```python
from build123d import *

# Parameters (mm, degrees)
F0_W     = 101.6
F0_H     = 50.8
F1_DEPTH = 25.4
F2_W     = 50.8
F2_H     = 12.7
F3_DEPTH = 25.401
F4_W     = 19.05
F4_H     = 12.7
F5_DEPTH = 25.401
F6_R     = 6.35
F7_DEPTH = 50.801
F8_DEPTH = 50.801


with BuildPart() as f1:
    # F0 (on Front) → F1 (new body)
    with BuildSketch(Plane.XZ):
        Rectangle(F0_W, F0_H)
    extrude(amount=F1_DEPTH)

    # F2 (on face) → F3 (cut, through all)
    with BuildSketch(Plane.XZ.offset(25.4)):
        with Locations((0, 19.05)):
            Rectangle(F2_W, F2_H)
    extrude(amount=-F3_DEPTH, mode=Mode.SUBTRACT)

    # F4 (on Front) → F5 (cut, through all)
    with BuildSketch(Plane.XZ):
        with Locations((41.358551, -19.152182)):
            Rectangle(F4_W, F4_H)
    extrude(amount=F5_DEPTH, mode=Mode.SUBTRACT)

    # F6 (on Right) → F7 (cut, through all)
    with BuildSketch(Plane.YZ):
        with Locations((-13.521904, 0.013301)):
            Circle(F6_R)
    extrude(amount=-F7_DEPTH, mode=Mode.SUBTRACT)

    # F6 (on Right) → F8 (cut, through all)
    with BuildSketch(Plane.YZ):
        with Locations((-13.521904, 0.013301)):
            Circle(F6_R)
    extrude(amount=F8_DEPTH, mode=Mode.SUBTRACT)


solid = f1.part
```
Can you work these out from the model? Positions are in its coordinate system, mm. A direction names the side the tool comes from. Round coordinates to 2 decimals unless told otherwise and drop trailing zeros. Loops run counter-clockwise (first coordinate to the right, second up) from the corner with the lowest first, then second, coordinate; pieces in that order, holes last. Notation, with made-up numbers: (84, -35.75) -> (113, -35.75) arc R26 ccw to (113, -1.75) -> close; hole circle Ø3 at (80.25, 68.25). An arc over 180 degrees is marked (long way). Answer in a Markdown table with one row per item.
Item 1: On a 3-axis mill with a long thin cutter (end or side, diameter ignored), from which of +Z, -Z, +X, -X, +Y, -Y can I reach the whole of each face in a straight line? I mean faces 5 (the flat face through (38, -13, 25.4)), 6 (the flat face through (25.4, -13, 19)), 7 (the flat face through (41, -13, -12.802)). Say none if no direction works.
Answer block:
| item | result |
|---|---|
| face 5 | +Z, +X, -X, +Y, -Y |
| face 6 | +Z, +Y, -Y |
| face 7 | -Z, +X, +Y, -Y |
Item 2: If I drill on probe 1 along X at (y, z) = (-20.75, 19.5); probe 2 along Z at (x, y) = (-21, -15.75); probe 3 along Z at (x, y) = (40.5, -16), over which ranges is the centre line in solid material (lowest first)?
Answer block:
| item | result |
|---|---|
| probe 1 | -50.8 to -25.4, 25.4 to 50.8 |
| probe 2 | -25.4 to -5.93, 5.96 to 12.7 |
| probe 3 | -12.8 to -5.83, 5.86 to 25.4 |
Item 3: Suppose I cut it at C-C, the plane x = 33.5. List the corners of the cut face in (y, z) for me, plus the area to 3 significant figures.
Answer block:
| item | result |
|---|---|
| outline | (-25.4, -12.8) -> (0, -12.8) -> (0, 25.4) -> (-25.4, 25.4) -> close; hole circle Ø12.7 at (-13.52, 0.01) |
| area | 844 mm² |
Item 4: We'd pull the mould along X, two halves only. Please class faces 1 (the flat face through (-50.8, -7, 0)), 2 (the flat face through (-1, -25.4, 0)), 3 (the flat face through (31.834, -13, -19)), 4 (the flat face through (0, -13, 12.7)): released by +X, released by -X, zero draft, split by the parting line, or undercut.
Answer block:
| item | result |
|---|---|
| face 1 | released by -X |
| face 2 | zero draft |
| face 3 | released by +X |
| face 4 | undercut |
Item 5: Suppose I cut it at A-A, the plane z = 14. List the corners of the cut face in (x, y) for me, plus the area to 3 significant figures.
Answer block:
| item | result |
|---|---|
| outline | (-50.8, -25.4) -> (-25.4, -25.4) -> (-25.4, 0) -> (-50.8, 0) -> close; (25.4, -25.4) -> (50.8, -25.4) -> (50.8, 0) -> (25.4, 0) -> close |
| area | 1,290 mm² |
Item 6: Suppose I cut it at B-B, the plane y = -17. List the corners of the cut face in (x, z) for me.
Answer block:
| item | result |
|---|---|
| outline | (-50.8, -25.4) -> (31.83, -25.4) -> (31.83, -12.8) -> (50.8, -12.8) -> (50.8, -5.3) -> (-50.8, -5.3) -> close; (-50.8, 5.33) -> (50.8, 5.33) -> (50.8, 25.4) -> (25.4, 25.4) -> (25.4, 12.7) -> (-25.4, 12.7) -> (-25.4, 25.4) -> (-50.8, 25.4) -> close |
Item 7: Suppose I cut it at D-D, the plane y = -6. List the corners of the cut face in (x, z) for me, plus the area to 3 significant figures.
Answer block:
| item | result |
|---|---|
| outline | (-50.8, -25.4) -> (31.83, -25.4) -> (31.83, -12.8) -> (50.8, -12.8) -> (50.8, 25.4) -> (25.4, 25.4) -> (25.4, 12.7) -> (-25.4, 12.7) -> (-25.4, 25.4) -> (-50.8, 25.4) -> close |
| area | 4,280 mm² |
Item 8: Will these pins go through, and if not, where does the flat tip stop? P1, Ø1.5, axis at x = 8, z = -10.5, coming from the +Y side; P2, Ø12, axis at x = -1, y = -6, coming from the +Z side; P3, Ø1.5, axis at y = -8, z = -14.5, coming from the +X side; P4, Ø5.5, axis at x = 39.5, y = -13.5, coming from the -Z side.
Answer block:
| item | result |
|---|---|
| P1 | y = 0 |
| P2 | z = 12.7 |
| P3 | x = 31.83 |
| P4 | z = -12.8 |
